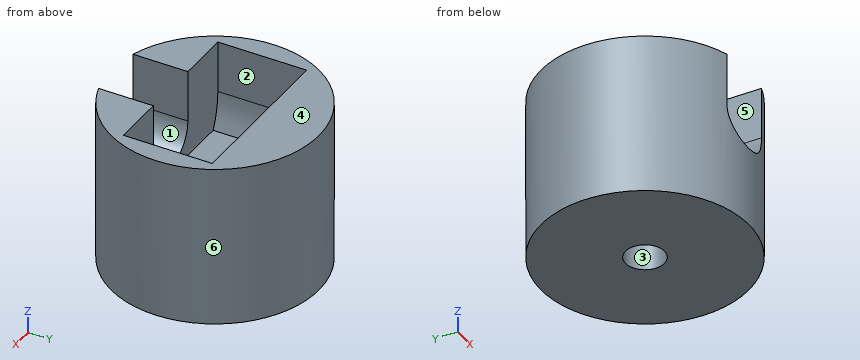
from build123d import *

# Parameters (mm, degrees)
SKETCH1_R               = 16
SKETCH1_R_2             = 3
BOSS_EXTRUDE1_DEPTH     = 25
CUT_EXTRUDE1_DEPTH      = 6.85
CUT_EXTRUDE2_REACH      = 35.719
CUT_EXTRUDE2_END_RADIUS = 16


with BuildPart() as part:
    # Sketch1 → Boss-Extrude1 (new body)
    with BuildSketch(Plane.XY):
        Circle(SKETCH1_R)
        Circle(SKETCH1_R_2, mode=Mode.SUBTRACT)
    extrude(amount=BOSS_EXTRUDE1_DEPTH)

    # Sketch2 → Cut-Extrude1 (cut, symmetric)
    with BuildSketch(Plane(origin=(0, 0, 0), x_dir=(1, 0, 0), z_dir=(0, 1, 0))):
        with BuildLine():
            Line((-11.589650556, -11.45), (11.589650556, -11.45))
            ThreePointArc((11.589650556, -11.45), (12.530951872, -14.154346265), (12.85, -17))
            Line((12.85, -17), (12.85, -25))
            Line((12.85, -25), (-12.85, -25))
            Line((-12.85, -25), (-12.85, -17))
            ThreePointArc((-12.85, -17), (-12.530951872, -14.154346265), (-11.589650556, -11.45))
        make_face()
    extrude(amount=CUT_EXTRUDE1_DEPTH, both=True, mode=Mode.SUBTRACT)

    # Cut-Extrude2: up to this cylinder (the profile starts inside it)
    cut_extrude2_end = Plane(origin=(0, 0, 19.107252), z_dir=(0, 0, -1)) * Cylinder(CUT_EXTRUDE2_END_RADIUS, 104.438, mode=Mode.PRIVATE)
    # Sketch3 → Cut-Extrude2 (cut, up to the surface)
    with BuildSketch(Plane(origin=(0, 0, 0), x_dir=(1, 0, 0), z_dir=(0, 1, 0)), mode=Mode.PRIVATE) as cut_extrude2_sk1:
        with BuildLine():
            Line((-4.7, -17), (-4.7, -25))
            Line((-4.7, -25), (4.7, -25))
            Line((4.7, -25), (4.7, -17))
            ThreePointArc((4.7, -17), (0, -12.3), (-4.7, -17))
        make_face()
    cut_extrude2_tool1 = extrude(cut_extrude2_sk1.sketch, amount=-CUT_EXTRUDE2_REACH, mode=Mode.PRIVATE) & cut_extrude2_end
    add(cut_extrude2_tool1.solids().sort_by_distance((0, 0, 19.107252))[0], mode=Mode.SUBTRACT)


solid = part.part
Model file for the job. Use its own axes, mm. Face numbers are marked on the shaded views. A direction names the side the tool comes from. Give positions to 0.01 mm unless a question says otherwise; leave off trailing zeros. Order: outer loops, then holes, each group sorted by start corner. A loop starts at its lowest first (then second) coordinate and runs counter-clockwise, first axis right, second up. Notation, with made-up numbers: (77, 63) - (97, 63) arc R23 ccw to (97, 92) - close; hole circle Ø4 at (-10.75, 76). An arc over 180 degrees is marked (long way). Return JSON: item names as keys, results as strings.
1) Pull direction X, two halves, no side cores. Call the marked faces 4, 5 and 6: pulls with the +X half, pulls with the -X half, needs draft (parallel to the pull), parting line crosses it, or undercut.
Geometry says:
{"face 4": "needs draft", "face 5": "undercut", "face 6": "parting line crosses it"}
2) Cut at B-B, the plane x = 0. Give the cut face in (y, z), plus the area to 3 significant figures.
Geometry says:
{"outline": "(-16, 0) - (-3, 0) - (-3, 11.45) - (-6.85, 11.45) - (-6.85, 12.3) - (-16, 12.3) - close; (3, 0) - (16, 0) - (16, 25) - (6.85, 25) - (6.85, 11.45) - (3, 11.45) - close", "area": "429 mm²"}
3) Cut at C-C, the plane z = 7.5. Give the cut face in (x, y).
Geometry says:
{"outline": "circle Ø32 at (0, 0); hole circle Ø6 at (0, 0)"}
4) Probe line 1 (X direction, y = 0, z = 8.5); line 2 (Z direction, x = 7, y = 5.5). List the from-to ranges inside material, lowest first. Write a range as from..to.
Geometry says:
{"line 1": "-16..-3, 3..16", "line 2": "0..11.45"}
5) 3-axis set-ups, long thin cutter, end or side, ignore diameter. For the marked faces 1, 2 and 3: which of +Z, -Z, +X, -X, +Y, -Y reach the whole face in a straight line?
Geometry says:
{"face 1": "+Z, -Y", "face 2": "+Z", "face 3": "+Z, -Z"}
6) Flat gauge pins, fed straight in: P1, Ø9, axis at y = -10.5, z = 22, coming from the +X side; P2, Ø1.5, axis at x = 9.5, y = 1.5, coming from the +Z side; P3, Ø5, axis at x = -11, z = 21.5, coming from the +Y side. Where does each tip first touch, or does it go through?
Geometry says:
{"P1": "x = 14.83", "P2": "z = 11.45", "P3": "y = 13.56"}
7) Cut at D-D, the plane y = 4.5. Give the cut face in (x, z), plus the area to 3 significant figures.
Geometry says:
{"outline": "(-15.35, 0) - (15.35, 0) - (15.35, 25) - (12.85, 25) - (12.85, 17) arc R12.85 cw to (11.59, 11.45) - (-11.59, 11.45) arc R12.85 cw to (-12.85, 17) - (-12.85, 25) - (-15.35, 25) - close", "area": "424 mm²"}
8) Cut at A-A, the plane y = 0. Give the cut face in (x, z).
Geometry says:
{"outline": "(-16, 0) - (-3, 0) - (-3, 11.45) - (-11.59, 11.45) arc R12.85 cw to (-12.85, 17) - (-12.85, 25) - (-16, 25) - close; (3, 0) - (16, 0) - (16, 25) - (12.85, 25) - (12.85, 17) arc R12.85 cw to (11.59, 11.45) - (3, 11.45) - close"}
